The model under review builds one solid part; all positions refer to its coordinate system, in mm. A direction names the side the tool comes from. Coordinates: 2 decimals unless noted, no trailing zeros. Write each loop counter-clockwise with the first axis right and the second up, starting at its lowest first coordinate (ties: lowest second). Pieces come first, ordered by that corner, then holes.
1) For line 1 (Z direction, x = 6, y = 1.75); line 2 (Y direction, x = 9.5, z = 14.25); line 3 (X direction, y = -4.5, z = 11.25), list the stretches that pass through material, from the lowest coordinate up.
2) Add section A-A, the plane y = 0. State the section outline as (x, z) points (3 decimals), then the cut area to 3 significant figures.
3) Add section B-B, the plane z = 5. State the section outline as (x, y) points (3 decimals).
4) For P1, Ø4, axis at y = 6.5, z = 16, coming from the +X side; P2, Ø6, axis at y = -6, z = 12, coming from the -X side; P3, Ø12, axis at y = 0.5, z = 17.5, coming from the +X side (3 decimals); P4, Ø8, axis at x = 17.5, z = 7, coming from the +Y side, all flat-tipped, find the tip position at first contact; note any pin that passes through.
5) Mouldability with a two-part tool opening along X and no side actions: class faces 3 (the cylindrical face through (-0.75, 0.03, -1.43)), 4 (the cylindrical face through (22.45, 4.19, 10.63)), 5 (the flat face through (9, -3, 21.44)) as released by +X, released by -X, zero draft, split by the parting line, or undercut.
6) Machinability: for faces 1 (the flat face through (18, 0, -3)), 2 (the cylindrical face through (17.54, 0.03, -1.43)), which of the approach directions +Z, -Z, +X, -X, +Y, -Y give a long, thin tool a straight path to every point of the face, cutting with its end or side? Answer none if there is none.
from build123d import *

# Parameters (mm, degrees)
SKETCH001_R       = 0.75
PAD001_DEPTH      = 10.67
PAD001_DEPTH_BACK = 3.5
SKETCH_R          = 13.95
SKETCH_R_2        = 1.46
PAD_DEPTH         = 21.34
FILLET_R          = 0.5


with BuildPart() as pad001:
    # Sketch001 → Pad001 (new body, two sides)
    with BuildSketch(Plane.XY.offset(0.5)) as pad001_sk:
        Circle(SKETCH001_R)
        with Locations((18.29, 0)):
            Circle(SKETCH001_R)
    extrude(amount=PAD001_DEPTH)
    extrude(pad001_sk.sketch, amount=-PAD001_DEPTH_BACK)


with BuildPart() as obj1:
    # Sketch → Pad (new body)
    with BuildSketch(Plane.XY.offset(0.1)):
        with Locations((9.145, 0)):
            Circle(SKETCH_R)
        with Locations((9.145, 0)):
            Circle(SKETCH_R_2, mode=Mode.SUBTRACT)
    extrude(amount=PAD_DEPTH)

    # Fillet
    fillet_edges = [obj1.edges().sort_by_distance(p)[0] for p in [
        (7.685, 0, 21.44),
        (-4.805, 0, 21.44),
        (-4.805, 0, 0.1),
    ]]
    fillet(fillet_edges, radius=FILLET_R)

    # obj1: union Pad001
    add(pad001.part)


solid = obj1.part
Geometry results:
1. line 1: z = 0.1 to 21.44
1. line 2: y = -13.95 to -1.42, 1.42 to 13.95
1. line 3: x = -4.06 to 22.35
2. outline: (-4.805, 0.6) arc R0.5 ccw to (-4.305, 0.1) - (-0.75, 0.1) - (-0.75, -3) - (0.75, -3) - (0.75, 0.1) - (7.685, 0.1) - (7.685, 20.94) arc R0.5 ccw to (7.185, 21.44) - (-4.305, 21.44) arc R0.5 ccw to (-4.805, 20.94) - close; (10.605, 0.1) - (17.54, 0.1) - (17.54, -3) - (19.04, -3) - (19.04, 0.1) - (22.595, 0.1) arc R0.5 ccw to (23.095, 0.6) - (23.095, 20.94) arc R0.5 ccw to (22.595, 21.44) - (11.105, 21.44) arc R0.5 ccw to (10.605, 20.94) - close
2. area: 542 mm2
3. outline: circle Ø27.9 at (9.145, 0); hole circle Ø2.92 at (9.145, 0)
4. P1: stops at x = 22.35
4. P2: stops at x = -4.48
4. P3: stops at x = 23.095
4. P4: stops at y = 13.25
5. face 3: undercut
5. face 4: split by the parting line
5. face 5: zero draft
6. face 1: -Z, +X, -X, +Y, -Y
6. face 2: -Z
